Input: part model. Units: mm. Frame: model coordinates. A direction names the side the tool comes from. Round coordinates to 2 decimals unless told otherwise and drop trailing zeros. Loops run counter-clockwise (first coordinate to the right, second up) from the corner with the lowest first, then second, coordinate; pieces in that order, holes last. Notation, with made-up numbers: (29, -23) -> (68, -23) arc R21 cw to (68, -4) -> close; hole circle Ø2 at (-31.5, 29). An arc over 180 degrees is marked (long way). One line per question, with ' | ' between items. Start each with the question number.
Q1. Mould query, pull axis X, two halves, no side actions, for faces 5 (the face through (38.5, 44, 14)), 6 (the face through (-1, -51, 26)), 7 (the face through (0, 12.064, 12)). Classes: pulls with the +X half, pulls with the -X half, needs draft (parallel to the pull), parting line crosses it, or undercut.
Q2. Cut plane D-D on x = 31.5. Return loops of the section in (y, z), and give its area (3 significant figures).
Q3. Cut plane C-C on y = 27. Return loops of the section in (x, z).
Q4. Contact query for flat-ended pins moving along their axis: P1, Ø6, axis at y = -2.5, z = 4, coming from the -X side (3 decimals); P2, Ø4, axis at x = 1.5, z = 13, coming from the +Y side; P3, Ø2, axis at y = -30, z = 12, coming from the +X side (3 decimals). Output: stop coordinate, or through.
Q5. Cut plane A-A on z = 14.5. Return loops of the section in (x, y), and give its area (3 significant figures).
Q6. Material intervals for L1, parallel to Y at x = 26, z = 1.75; L2, parallel to Y at x = 28.5, z = 20.5 (3 decimals); L3, parallel to Y at x = -13.5, z = 26.5, sorted ascending.
Q7. Access query for faces 1 (the face through (0, 0, 25)), 2 (the face through (-7.535, 0.14, 12.325)), 3 (the face through (0, 2, 10)), 4 (the face through (0, 44, 12)). Directions: +Z, -Z, +X, -X, +Y, -Y. A direction counts if a zero-diameter tool reaches every point of the face in a straight line with its end or side. Return the directions, or none.
Q8. Cut plane B-B on z = 2.5. State how many separate pieces and enclosed holes the cut face has, and give its area (3 significant figures).
from build123d import *

# Parameters (mm, degrees)
F1_DEPTH   = 25
F2_DEPTH   = 10
F0_W       = 77
F0_H       = 3
F3_DEPTH   = 29
F4_SIZE2   = 3
F4_SIZE    = 25
F4_2_SIZE2 = 3
F4_2_SIZE  = 25
F5_SIZE    = 1


with BuildPart() as f1:
    # F0 (on Top) → F1 (new body)
    with BuildSketch(Plane.XY):
        Polygon((-38.5, -38), (-38.5, -48), (38.5, -48), (38.5, -38), (5, -10), (0.4688645929, -11.4259910617), (34.5, -39.8699251333), (34.5, -44), (-34.5, -44), (-34.5, -39.8699251333), (-0.5114898408, -11.4616181345), (-5, -10), align=None)
        Polygon((-10, 10), (-5, -10), (-0.5114898408, -11.4616181345), (0.4688645929, -11.4259910617), (5, -10), (10, 10), (6.3927714964, 12.0635084879), (-6.3927714964, 12.0635084879), align=None)
        Polygon((5.520849137, 8.1635084879), (1.7461076086, -6.9354576256), (-0.0650228365, -7.5054374638), (-1.7399680433, -6.9600158871), (-5.520849137, 8.1635084879), align=None, mode=Mode.SUBTRACT)
        Polygon((-38.5, 38), (-10, 10), (-6.3927714964, 12.0635084879), (-34.5, 39.6776277196), (-34.5, 44), (34.5, 44), (34.5, 39.6776277196), (6.3927714964, 12.0635084879), (10, 10), (38.5, 38), (38.5, 48), (-38.5, 48), align=None)
        Polygon((-0.0650228365, -7.5054374638), (1.7461076086, -6.9354576256), (5.520849137, 8.1635084879), (-5.520849137, 8.1635084879), (-1.7399680433, -6.9600158871), align=None)
    extrude(amount=F1_DEPTH)

    # F0 (on Top) → F2 (cut)
    with BuildSketch(Plane.XY):
        Polygon((-0.0650228365, -7.5054374638), (1.7461076086, -6.9354576256), (5.520849137, 8.1635084879), (-5.520849137, 8.1635084879), (-1.7399680433, -6.9600158871), align=None)
    extrude(amount=F2_DEPTH, mode=Mode.SUBTRACT)

    # F0 (on Top) → F3 (join)
    with BuildSketch(Plane.XY):
        with Locations((0, -49.5)):
            Rectangle(F0_W, F0_H)
        with Locations((0, 49.5)):
            Rectangle(F0_W, F0_H)
    extrude(amount=F3_DEPTH)

    # F4
    f4_edges = [f1.edges().sort_by_distance(p)[0] for p in [
        (0, -51, 0),
    ]]
    f4_side = f1.faces().sort_by_distance((0, -51, 14.5))[0]
    chamfer(f4_edges, length=F4_SIZE, length2=F4_SIZE2, reference=f4_side)

    # F4#2
    f4_2_edges = [f1.edges().sort_by_distance(p)[0] for p in [
        (0, 51, 0),
    ]]
    f4_2_side = f1.faces().sort_by_distance((0, 51, 14.5))[0]
    chamfer(f4_2_edges, length=F4_2_SIZE, length2=F4_2_SIZE2, reference=f4_2_side)

    # F5
    f5_edges = [f1.edges().sort_by_distance(p)[0] for p in [
        (0, -51, 29),
        (0, 51, 29),
    ]]
    chamfer(f5_edges, length=F5_SIZE)


solid = f1.part
Results:
1) face 5: pulls with the +X half | face 6: needs draft | face 7: undercut
2) outline: (-51, 25) -> (-48, 0) -> (-44, 0) -> (-44, 25) -> (-48, 25) -> (-48, 29) -> (-50, 29) -> (-51, 28) -> close; (-37.36, 0) -> (-32.15, 0) -> (-32.15, 25) -> (-37.36, 25) -> close; (31.12, 0) -> (36.73, 0) -> (36.73, 25) -> (31.12, 25) -> close; (44, 0) -> (48, 0) -> (51, 25) -> (51, 28) -> (50, 29) -> (48, 29) -> (48, 25) -> (44, 25) -> close | area: 569 mm^2
3) outline: (-27.3, 0) -> (-21.6, 0) -> (-21.6, 25) -> (-27.3, 25) -> close; (21.6, 0) -> (27.3, 0) -> (27.3, 25) -> (21.6, 25) -> close
4) P1: x = -7.625 | P2: y = 49.8 | P3: x = 30.125
5) outline: (-38.5, -49.74) -> (38.5, -49.74) -> (38.5, -38) -> (5, -10) -> (10, 10) -> (38.5, 38) -> (38.5, 49.74) -> (-38.5, 49.74) -> (-38.5, 38) -> (-10, 10) -> (-5, -10) -> (-38.5, -38) -> close; hole (-34.5, -44) -> (34.5, -44) -> (34.5, -39.87) -> (0.47, -11.43) -> (-0.51, -11.46) -> (-34.5, -39.87) -> close; hole (-34.5, 39.68) -> (-6.39, 12.06) -> (6.39, 12.06) -> (34.5, 39.68) -> (34.5, 44) -> (-34.5, 44) -> close | area: 1,980 mm^2
6) L1: -48.21 to -44, -32.77 to -27.55, 25.72 to 31.33, 44 to 48.21 | L2: -50.46 to -44, -34.855 to -29.642, 28.175 to 33.783, 44 to 50.46 | L3: -51 to -48, 48 to 51
7) face 1: +Z, +X, -X | face 2: +Z, -Z, -X | face 3: -Z | face 4: +Z, -Z
8) separate pieces: 1 | enclosed holes: 3 | area: 1,640 mm^2
